Verification items for the finished model (mm, model axes). A direction names the side the tool comes from. Coordinates: 2 decimals unless noted, no trailing zeros. Loops run counter-clockwise (first coordinate to the right, second up) from the corner with the lowest first, then second, coordinate; pieces in that order, holes last. Notation, with made-up numbers: (83, 86.5) - (116, 86.5) arc R27 cw to (116, 112.5) - close; hole circle Ø10 at (-19.75, -1). An arc over 180 degrees is marked (long way). Answer as CSV lines item,"result". Start each with the question number.
1. Cross-section at C-C (y = 2.75). Enter the section's corners in (x, z) (3 decimals), plus the area to 3 significant figures.
2. Gauge pin test, flat ends, axial feed: P1, Ø6, axis at x = -7, y = 5, coming from the +Z side; P2, Ø6, axis at y = 5, z = 24.5, coming from the +X side; P3, Ø5, axis at y = 6.5, z = -11, coming from the -X side; P4, Ø5, axis at x = 10, z = 28, coming from the -Y side. Record the tip position at first contact, or that the pin passes through.
3. Cross-section at B-B (x = 0). Enter the section's corners in (y, z) (3 decimals).
4. Cross-section at D-D (x = 18). Enter the section's corners in (y, z).
5. Material ranges on line 1 (X direction, y = 2.85, z = 0) (3 decimals); line 2 (Z direction, x = 0, y = 3.2) (3 decimals); line 3 (X direction, y = 6.45, z = 0), recorded low to high. Write a range as [from, to].
6. Release check for a two-part mould opening along X. For faces 1 (the flat face through (-1, 0, -1)), 2 (the cylindrical face through (-22.37, 2.46, -0.95)), 3 (the cylindrical face through (-41.265, 4.93, 31.641)) record: pulls with the +X half, pulls with the -X half, needs draft (parallel to the pull), parting line crosses it, or undercut.
7. Set-up check for faces 4 (the cylindrical face through (-0.69, 2.46, 34.85)), 5 (the flat face through (-1, 5, -1)): record each of +Z, -Z, +X, -X, +Y, -Y from which the full face is reachable in a straight line by a thin tool's end or side.
8. Cross-section at A-A (z = 0). Enter the section's corners in (x, y) (3 decimals), plus the area to 4 significant figures.
```python
from build123d import *

# Parameters (mm, degrees)
SKETCH1_R           = 52
SKETCH1_R_2         = 3.175
SKETCH1_R_3         = 2.38
BOSS_EXTRUDE1_DEPTH = 5
SKETCH2_R           = 52
SKETCH2_R_2         = 49.6
BOSS_EXTRUDE2_DEPTH = 5


with BuildPart() as part:
    # Sketch1 → Boss-Extrude1 (new body)
    with BuildSketch(Plane(origin=(0, 0, 0), x_dir=(1, 0, 0), z_dir=(0, 1, 0))):
        Circle(SKETCH1_R)
        with Locations((25.4, 0)):
            Circle(SKETCH1_R_2, mode=Mode.SUBTRACT)
        with Locations((0, 31.75)):
            Circle(SKETCH1_R_2, mode=Mode.SUBTRACT)
        with Locations((-25.4, 0)):
            Circle(SKETCH1_R_2, mode=Mode.SUBTRACT)
        with Locations((0, -31.75)):
            Circle(SKETCH1_R_2, mode=Mode.SUBTRACT)
        with Locations((18, 18)):
            Circle(SKETCH1_R_3, mode=Mode.SUBTRACT)
    extrude(amount=BOSS_EXTRUDE1_DEPTH)

    # Sketch2 → Boss-Extrude2 (add)
    with BuildSketch(Plane(origin=(0, 5, 0), x_dir=(1, 0, 0), z_dir=(0, 1, 0))):
        Circle(SKETCH2_R)
        Circle(SKETCH2_R_2, mode=Mode.SUBTRACT)
    extrude(amount=BOSS_EXTRUDE2_DEPTH)


solid = part.part
```
Values follow:
1,outline,"circle Ø104 at (0, 0); hole circle Ø6.35 at (-25.4, 0); hole circle Ø6.35 at (0, -31.75); hole circle Ø6.35 at (0, 31.75); hole circle Ø4.76 at (18, -18); hole circle Ø6.35 at (25.4, 0)"
1,area,"8,350 mm²"
2,P1,"stops at z = 51.85"
2,P2,"stops at x = 47.35"
2,P3,"stops at x = -51.3"
2,P4,"stops at y = 0"
3,outline,"(0, -52) - (10, -52) - (10, -49.6) - (5, -49.6) - (5, -34.925) - (0, -34.925) - close; (0, -28.575) - (5, -28.575) - (5, 28.575) - (0, 28.575) - close; (0, 34.925) - (5, 34.925) - (5, 49.6) - (10, 49.6) - (10, 52) - (0, 52) - close"
4,outline,"(0, -48.79) - (10, -48.79) - (10, -46.22) - (5, -46.22) - (5, -20.38) - (0, -20.38) - close; (0, -15.62) - (5, -15.62) - (5, 46.22) - (10, 46.22) - (10, 48.79) - (0, 48.79) - close"
5,line 1,"x = [-52, -28.575], [-22.225, 22.225], [28.575, 52]"
5,line 2,"z = [-52, -34.925], [-28.575, 28.575], [34.925, 52]"
5,line 3,"x = [-52, -49.6], [49.6, 52]"
6,face 1,"needs draft"
6,face 2,"undercut"
6,face 3,"parting line crosses it"
7,face 4,"+Y, -Y"
7,face 5,"+Y"
8,outline,"(-52, 0) - (-28.575, 0) - (-28.575, 5) - (-49.6, 5) - (-49.6, 10) - (-52, 10) - close; (-22.225, 0) - (22.225, 0) - (22.225, 5) - (-22.225, 5) - close; (28.575, 0) - (52, 0) - (52, 10) - (49.6, 10) - (49.6, 5) - (28.575, 5) - close"
8,area,"480.5 mm²"
